Here's the drawing with two shaded views (mm, measured from the low corner). I have some questions. Coordinates: 2 decimals unless noted, no trailing zeros. Loops run counter-clockwise (first coordinate to the right, second up) from the corner with the lowest first, then second, coordinate; pieces in that order, holes last. Notation, with made-up numbers: (73.25, -17.75) - (84.25, -17.75) arc R16 cw to (84.25, -5.75) - close; hole circle Ø6 at (33.5, 85). An arc over 180 degrees is marked (long way). One line per item, written item: value. Start each with the question number.
(1) If we section it at A-A on x = 55: Write out the boundary of the cut face in (y, z).
(2) If I drill on line 1 along Z through (x, y) = (78, 0.7); line 2 along X through (y, z) = (0.45, 54.5); line 3 along X through (y, z) = (1.1, 5.5), over which ranges is the centre line in solid material (lowest first)? Write a range as from..to.
(3) I'm going to push flat-ended pins straight in: P1, Ø0.6, axis at y = 2.5, z = 17, coming from the -X side; P2, Ø1.5, axis at y = 1, z = 22, coming from the -X side; P3, Ø2, axis at x = 28.5, y = 2.5, coming from the -Z side; P4, Ø0.6, axis at y = 2, z = 30.5, coming from the +X side. Where does each tip first touch, or does it pass through?
(4) If we section it at B-B on z = 15: Write out the boundary of the cut face in (x, y).
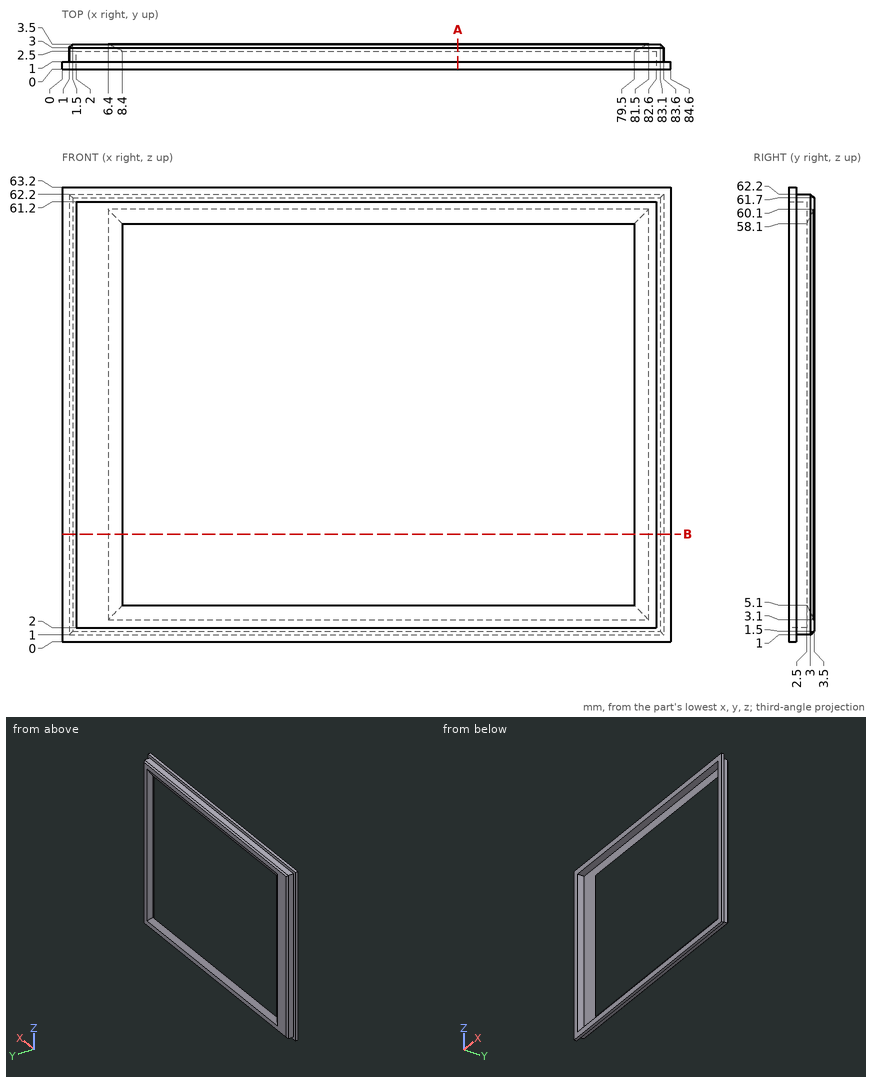
Values:
1. outline: (0, 0) - (1, 0) - (1, 1) - (3, 1) - (3.5, 1.5) - (3.5, 3.1) - (2.5, 5.1) - (2.5, 2) - (0, 2) - close; (0, 61.2) - (2.5, 61.2) - (2.5, 58.1) - (3.5, 60.1) - (3.5, 61.7) - (3, 62.2) - (1, 62.2) - (1, 63.2) - (0, 63.2) - close
2. line 1: z = 0..2, 61.2..63.2
2. line 2: x = 0..2, 82.6..84.6
2. line 3: x = 1..2, 82.6..83.6
3. P1: stops at x = 1
3. P2: stops at x = 0
3. P3: stops at z = 1
3. P4: stops at x = 83.6
4. outline: (0, 0) - (2, 0) - (2, 2.5) - (8.4, 2.5) - (6.4, 3.5) - (1.5, 3.5) - (1, 3) - (1, 1) - (0, 1) - close; (79.5, 2.5) - (82.6, 2.5) - (82.6, 0) - (84.6, 0) - (84.6, 1) - (83.6, 1) - (83.6, 3) - (83.1, 3.5) - (81.5, 3.5) - close
